from build123d import *

# Parameters (mm, degrees)
SKETCH_1_R               = 9
EXTRUDE_1_DEPTH          = 5
EXTRUDE_START            = -5
EXTRUDE_2_DEPTH          = 5
PATTERN_CIRCULAR_1_COUNT = 10
CUT_EXTRUDE_1_REACH      = 16.88
SKETCH_3_R               = 2.1


with BuildPart() as part:
    # 草图1 → 凸台-拉伸1 (new body)
    with BuildSketch(Plane(origin=(0, 0, 0), x_dir=(1, 0, 0), z_dir=(0, 1, 0))):
        with Locations(Location((0, 0, 0), (0, 0, 270))):
            Circle(SKETCH_1_R)
        with BuildLine():
            Line((-1.161895004, 1.1), (1.161895004, 1.1))
            ThreePointArc((1.161895004, 1.1), (0, -1.6), (-1.161895004, 1.1))
        make_face(mode=Mode.SUBTRACT)
    extrude(amount=EXTRUDE_1_DEPTH)

    # 草图2 → 凸台-拉伸2 (add)
    with BuildSketch(Plane(origin=(0, 5, 0), x_dir=(1, 0, 0), z_dir=(0, 1, 0)).offset(EXTRUDE_START)):
        with BuildLine():
            Line((1.5, 8.874119675), (1, 10))
            Line((1, 10), (-1, 10))
            Line((-1, 10), (-1.5, 8.874119675))
            ThreePointArc((-1.5, 8.874119675), (0, 9), (1.5, 8.874119675))
        make_face()
    extrude_2 = extrude(amount=EXTRUDE_2_DEPTH)

    # 阵列(圆周)1: 凸台-拉伸2 ×10 about axis
    pattern_circular_1_axis = Axis((0, 0, 0), (0, 1, 0))
    for i in range(1, PATTERN_CIRCULAR_1_COUNT):
        add(extrude_2.rotate(pattern_circular_1_axis, i * 360 / PATTERN_CIRCULAR_1_COUNT))

    # 草图3 → 切除-拉伸1 (cut, up to next)
    with BuildSketch(Plane(origin=(0, 5, 0), x_dir=(1, 0, 0), z_dir=(0, 1, 0)), mode=Mode.PRIVATE) as cut_extrude_1_sk1:
        with Locations(Location((0, 4.5, 0), (0, 0, 270))):
            Circle(SKETCH_3_R)
    cut_extrude_1_tool1 = extrude(cut_extrude_1_sk1.sketch, amount=-CUT_EXTRUDE_1_REACH, mode=Mode.PRIVATE) & part.part
    # 草图3 → 切除-拉伸1 (cut, up to next)
    with BuildSketch(Plane(origin=(0, 5, 0), x_dir=(1, 0, 0), z_dir=(0, 1, 0)), mode=Mode.PRIVATE) as cut_extrude_1_sk2:
        with Locations(Location((0, -4.5, 0), (0, 0, 270))):
            Circle(SKETCH_3_R)
    cut_extrude_1_tool2 = extrude(cut_extrude_1_sk2.sketch, amount=-CUT_EXTRUDE_1_REACH, mode=Mode.PRIVATE) & part.part
    add(cut_extrude_1_tool1.solids().sort_by_distance((0, 5, -4.5))[0], mode=Mode.SUBTRACT)
    add(cut_extrude_1_tool2.solids().sort_by_distance((0, 5, 4.5))[0], mode=Mode.SUBTRACT)


solid = part.part
The listing builds one solid part. Answer for the finished solid, in the listing's coordinates (mm). A direction names the side the tool comes from. Give positions to 0.01 mm unless a question says otherwise; leave off trailing zeros. Order: outer loops, then holes, each group sorted by start corner. A loop starts at its lowest first (then second) coordinate and runs counter-clockwise, first axis right, second up. Notation, with made-up numbers: (40, 41) - (90, 41) arc R24 ccw to (90, 61) - close; hole circle Ø10 at (21.5, 7.5). An arc over 180 degrees is marked (long way). Answer as CSV lines item,"result".
Q1. A cutting plane is placed at C-C, the plane y = 4.5. Count the separate pieces of the cut face and the enclosed holes in it, and give its area (3 significant figures).
Answer key:
separate pieces,"1"
enclosed holes,"3"
area,"245 mm^2"
Q2. Determine the mould class of faces 6 (the face through (-6, 2, 8)), 7 (the face through (-4.528, 2.465, -8.365)), 8 (the face through (0, 2, -1.1)) for opening direction Z: pulls with the +Z half, pulls with the -Z half, needs draft (parallel to the pull), parting line crosses it, or undercut.
Answer key:
face 6,"pulls with the +Z half"
face 7,"pulls with the -Z half"
face 8,"undercut"
Q3. Which of the six approach directions +Z, -Z, +X, -X, +Y, -Y give full straight-line access (tool end or side, diameter ignored) to faces 1 (the face through (-9.368, 2.465, -1.733)), 2 (the face through (9.355, 2.465, -1.722)), 3 (the face through (-4.54, 2.46, 8.37)), 4 (the face through (0, 2, 10)), 5 (the face through (2.799, 2.465, -8.554))?
Answer key:
face 1,"-X, +Y, -Y"
face 2,"+X, +Y, -Y"
face 3,"+Z, +Y, -Y"
face 4,"+Z, +X, -X, +Y, -Y"
face 5,"-Z, +Y, -Y"
Q4. A cutting plane is placed at A-A, the plane z = 0. Determine the outline of the cut face in (x, y), and give its area (3 significant figures).
Answer key:
outline,"(-9, 0) - (-1.6, 0) - (-1.6, 5) - (-9, 5) - close; (1.6, 0) - (9, 0) - (9, 5) - (1.6, 5) - close"
area,"74.0 mm^2"
Q5. A cutting plane is placed at D-D, the plane z = -4.5. Determine the outline of the cut face in (x, y), and give its area (3 significant figures).
Answer key:
outline,"(-7.79, 0) - (-2.1, 0) - (-2.1, 5) - (-7.79, 5) - close; (2.1, 0) - (7.79, 0) - (7.79, 5) - (2.1, 5) - close"
area,"56.9 mm^2"
Q6. Straight lines are drawn through the part: L1, parallel to X at y = 4.5, z = -5.75; L2, parallel to X at y = 1.7, z = -4.5; L3, parallel to Z at x = -2.25, y = 0.3. For each, find the intervals that lie inside material, in ascending order.
Answer key:
L1,"x = -6.92 to -1.69, 1.69 to 6.92"
L2,"x = -7.79 to -2.1, 2.1 to 7.79"
L3,"z = -8.71 to 8.71"
Q7. Each of these flat-tipped pins is pushed along its axis until it touches: pin 1 Ø1.5 at (x, y) = (-6, 4.5) entering from +Z; pin 2 Ø1.5 at (x, y) = (-6, 1) entering from -Z; pin 3 Ø1 at (y, z) = (3.5, 1.5) entering from +X. Where does it stop, or does it pass through?
Answer key:
pin 1,"stops at z = 8.55"
pin 2,"stops at z = -8.55"
pin 3,"stops at x = 9.66"
Q8. A cutting plane is placed at B-B, the plane x = 0. Determine the outline of the cut face in (y, z).
Answer key:
outline,"(0, -10) - (5, -10) - (5, -6.6) - (0, -6.6) - close; (0, -2.4) - (5, -2.4) - (5, -1.1) - (0, -1.1) - close; (0, 1.6) - (5, 1.6) - (5, 2.4) - (0, 2.4) - close; (0, 6.6) - (5, 6.6) - (5, 10) - (0, 10) - close"
